Verification items for the finished model (mm, model axes). Face numbers are marked on the shaded views. A direction names the side the tool comes from. Give positions to 0.01 mm unless a question says otherwise; leave off trailing zeros. Write each loop counter-clockwise with the first axis right and the second up, starting at its lowest first coordinate (ties: lowest second). Pieces come first, ordered by that corner, then holes. Notation, with made-up numbers: (-39, -7.5) -> (-8, -7.5) arc R16 ccw to (-8, 22.5) -> close; hole circle Ø5 at (82.5, 18.25). An arc over 180 degrees is marked (long way). Use one line per item in the form item = value. Start each with the question number.
(1) Section check A-A, the plane x = 13. Record the cut outline in (y, z).
(2) Section check C-C, the plane y = 11. Record the cut outline in (x, z), plus the area to 3 significant figures.
(3) Release check for a two-part mould opening along Z. For the marked faces 1, 2 and 3 record: pulls with the +Z half, pulls with the -Z half, needs draft (parallel to the pull), parting line crosses it, or undercut.
(4) Set-up check for the marked faces 4 and 5: record each of +Z, -Z, +X, -X, +Y, -Y from which the full face is reachable in a straight line by a thin tool's end or side.
(5) Scan lines: L1, parallel to Z at x = 5, y = -5.5; L2, parallel to Z at x = -3, y = -10.75; L3, parallel to Z at x = 0.25, y = -7.5. Record each from-to range of solid material in increasing order.
(6) Depth check by flat-ended pin: pin 1 Ø4 at (x, y) = (-10, 2) entering from -Z; pin 2 Ø2.5 at (x, y) = (-11.5, 5.5) entering from -Z; pin 3 Ø5 at (x, z) = (4, -2) entering from +Y. Enter the tip coordinate at first touch or a pass-through.
(7) Section check B-B, the plane z = 7.75. Record the cut outline in (x, y).
from build123d import *

# Parameters (mm, degrees)
EXTRUDE_1_DEPTH     = 9.5
SKETCH_6_R          = 7
EXTRUDE_2_DEPTH     = 9.5
SWEEP_1_PITCH       = 4
REVOLVE_2_ANGLE     = 45
CHAMFER_1_SIZE      = 1
CUT_EXTRUDE_2_DEPTH = 0.4
SKETCH_13_R         = 2.5
CUT_EXTRUDE_3_DEPTH = 0.4
CUT_EXTRUDE_4_DEPTH = 0.4
SKETCH_14_W         = 5
SKETCH_14_H         = 5
CUT_EXTRUDE_5_DEPTH = 0.4


with BuildPart() as part:
    # 草图1 → 凸台-拉伸1 (new body)
    with BuildSketch(Plane.XY):
        Polygon((15, 0), (7.5, 12.990381057), (-7.5, 12.990381057), (-15, 0), (-7.5, -12.990381057), (7.5, -12.990381057), align=None)
    extrude(amount=EXTRUDE_1_DEPTH)

    # 草图6 → 凸台-拉伸2 (add)
    with BuildSketch(Plane(origin=(0, 0, 0), x_dir=(-1, 0, 0), z_dir=(0, 0, -1))):
        Circle(SKETCH_6_R)
    extrude(amount=EXTRUDE_2_DEPTH)

    # 扫描1: the profile of 草图8 profile screwed along a right-hand helix of 1.5 turns, 12 arcs to a turn; built about Z, then put on its axis
    sweep_1_z = Axis((0, 0, 0), (0, 0, 1))
    sweep_1_corners = [(6.9997, 0, 1.7503), (6.9997, 0, -1.7503), (8.5, 0, -0.25), (8.5, 0, 0.25)]
    with BuildLine(mode=Mode.PRIVATE) as sweep_1_profile:
        Line(sweep_1_corners[0], sweep_1_corners[1])
        Line(sweep_1_corners[1], sweep_1_corners[2])
        Line(sweep_1_corners[2], sweep_1_corners[3])
        Line(sweep_1_corners[3], sweep_1_corners[0])
    sweep_1_cap = Face(sweep_1_profile.wire())
    sweep_1_turn_angles = [0, 15, 30, 45, 60, 75, 90, 105, 120, 135, 150, 165, 180, 195, 210, 225, 240, 255, 270, 285, 300, 315, 330, 345, 360]
    sweep_1_turn_weights = [1, 0.9659258262890683, 1, 0.9659258262890683, 1, 0.9659258262890683, 1, 0.9659258262890683, 1, 0.9659258262890683, 1, 0.9659258262890683, 1, 0.9659258262890683, 1, 0.9659258262890683, 1, 0.9659258262890683, 1, 0.9659258262890683, 1, 0.9659258262890683, 1, 0.9659258262890683, 1]
    sweep_1_turn_rails = [Edge.make_bspline([Vector(p[0], p[1], 0).rotate(sweep_1_z, sweep_1_turn_angles[k]) / sweep_1_turn_weights[k] + Vector(0, 0, p[2] + SWEEP_1_PITCH * sweep_1_turn_angles[k] / 360) for k in range(25)], [0, 0, 0, 1, 1, 2, 2, 3, 3, 4, 4, 5, 5, 6, 6, 7, 7, 8, 8, 9, 9, 10, 10, 11, 11, 12, 12, 12], 2, sweep_1_turn_weights) for p in sweep_1_corners]
    sweep_1_turn_sides = [Face.make_surface_from_curves(sweep_1_turn_rails[p[0]], sweep_1_turn_rails[p[1]]) for p in [(0, 1), (1, 2), (2, 3), (3, 0)]]
    sweep_1_last_angles = [360, 375, 390, 405, 420, 435, 450, 465, 480, 495, 510, 525, 540]
    sweep_1_last_weights = [1, 0.9659258262890683, 1, 0.9659258262890683, 1, 0.9659258262890683, 1, 0.9659258262890683, 1, 0.9659258262890683, 1, 0.965925826289066, 1]
    sweep_1_last_rails = [Edge.make_bspline([Vector(p[0], p[1], 0).rotate(sweep_1_z, sweep_1_last_angles[k]) / sweep_1_last_weights[k] + Vector(0, 0, p[2] + SWEEP_1_PITCH * sweep_1_last_angles[k] / 360) for k in range(13)], [0, 0, 0, 1, 1, 2, 2, 3, 3, 4, 4, 5, 5, 6, 6, 6], 2, sweep_1_last_weights) for p in sweep_1_corners]
    sweep_1_last_sides = [Face.make_surface_from_curves(sweep_1_last_rails[p[0]], sweep_1_last_rails[p[1]]) for p in [(0, 1), (1, 2), (2, 3), (3, 0)]]
    sweep_1 = Plane(origin=(0, 0, -1.75), x_dir=(-1, 0, 0), z_dir=(0, 0, -1)) * Solid(Shell([*sweep_1_turn_sides, *sweep_1_last_sides, sweep_1_cap, sweep_1_cap.rotate(sweep_1_z, 540).moved(Location((0, 0, SWEEP_1_PITCH * 540 / 360)))]))
    add(sweep_1)

    # 草图9 → 旋转2 (revolve)
    with BuildSketch(Plane(origin=(0, 0, 0), x_dir=(1, 0, 0), z_dir=(0, 1, 0))):
        Polygon((7, 3.5), (7, 0), (8.5, 1.5), (8.5, 2), align=None)
    revolve(axis=Axis((0, 0, 0), (0, 0, 1)), revolution_arc=REVOLVE_2_ANGLE)

    # 倒角1
    chamfer_1_edges = [part.edges().sort_by_distance(p)[0] for p in [
        (-11.25, 6.495190528, 9.5),
        (-11.25, -6.495190528, 9.5),
        (0, -12.990381057, 9.5),
        (11.25, -6.495190528, 9.5),
        (11.25, 6.495190528, 9.5),
        (11.25, -6.495190528, 0),
        (0, -12.990381057, 0),
        (-11.25, -6.495190528, 0),
        (-11.25, 6.495190528, 0),
        (0, 12.990381057, 0),
        (11.25, 6.495190528, 0),
        (0, 12.990381057, 9.5),
    ]]
    chamfer(chamfer_1_edges, length=CHAMFER_1_SIZE)

    # 草图11 → 切除-拉伸2 (cut)
    with BuildSketch(Plane(origin=(-11.25, -6.495190528, 0), x_dir=(0, 0, 1), z_dir=(-0.8660254037844389, -0.4999999999999995, 0))):
        Polygon((2.25, 0), (7.25, 2.886751346), (7.25, -2.886751346), align=None)
    extrude(amount=-CUT_EXTRUDE_2_DEPTH, mode=Mode.SUBTRACT)

    # 草图13 → 切除-拉伸3 (cut)
    with BuildSketch(Plane(origin=(11.25, -6.495190528, 0), x_dir=(0, 0, -1), z_dir=(0.8660254037844387, -0.5000000000000001, 0))):
        with Locations(Location((-4.75, 0, 0), (0, 0, 90))):
            Circle(SKETCH_13_R)
    extrude(amount=-CUT_EXTRUDE_3_DEPTH, mode=Mode.SUBTRACT)

    # 草图12 → 切除-拉伸4 (cut)
    with BuildSketch(Plane.XZ.offset(12.990381057)):
        Polygon((-2.5, 6.825735931), (2.075735931, 2.25), (2.5, 2.674264069), (-2.075735931, 7.25), align=None)
        Polygon((2.075735931, 7.25), (-2.5, 2.674264069), (-2.075735931, 2.25), (2.5, 6.825735931), align=None)
    extrude(amount=-CUT_EXTRUDE_4_DEPTH, mode=Mode.SUBTRACT)

    # 草图14 → 切除-拉伸5 (cut)
    with BuildSketch(Plane(origin=(-11.25, 6.495190528, 0), x_dir=(0, 0, 1), z_dir=(-0.8660254037844384, 0.5000000000000006, 0))):
        with Locations((4.75, 0)):
            Rectangle(SKETCH_14_W, SKETCH_14_H)
    extrude(amount=-CUT_EXTRUDE_5_DEPTH, mode=Mode.SUBTRACT)


solid = part.part
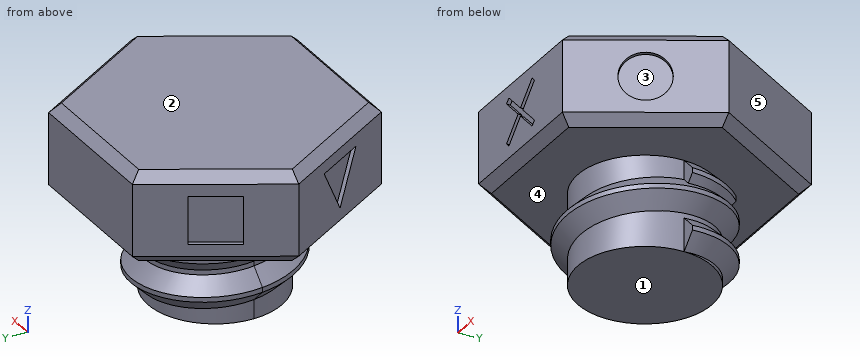
Completed:
q1.outline = (-3.46, 1) -> (-1.46, 0) -> (1.46, 0) -> (3.46, 1) -> (3.46, 8.5) -> (1.46, 9.5) -> (-1.46, 9.5) -> (-3.46, 8.5) -> close
q2.outline = (-8.65, 1) -> (-7.49, 0) -> (7.49, 0) -> (8.65, 1) -> (8.65, 8.5) -> (7.49, 9.5) -> (-7.49, 9.5) -> (-8.65, 8.5) -> close
q2.area = 162 mm²
q3.face_1 = pulls with the -Z half
q3.face_2 = pulls with the +Z half
q3.face_3 = undercut
q4.face_4 = none
q4.face_5 = +Z, -Z, +X, +Y
q5.L1 = -5.6 to -2.96, 0 to 9.5
q5.L2 = 0 to 9.5
q5.L3 = -5.98 to -3.48, 0 to 9.5
q6.pin_1 = -6.43
q6.pin_2 = 0
q6.pin_3 = 12.49
q7.outline = (-15, 0) -> (-7.5, -12.99) -> (7.5, -12.99) -> (15, 0) -> (7.5, 12.99) -> (-7.5, 12.99) -> close
